Could you check a few things on this model? Use its own coordinates, in mm. Give positions to 0.01 mm unless a question says otherwise; leave off trailing zeros.
1. Imagine slicing it at A-A (z = 1.9). Count the separate pieces of the cut face and the enclosed holes in it, plus the area to 3 significant figures.
2. I need wall thicknesses on line 1 along Y through (x, z) = (-120, 2.35); line 2 along Y through (x, z) = (-25.5, 1.45); line 3 along Y through (x, z) = (-93.5, 1). Which ranges of each line are inside material? Lowest first, please.
3. Thinking about a two-plate mould opening in X: for faces 1 (the cylindrical face through (-124.305, -1.532, 1.479)), 2 (the flat face through (-2, 14, 0)), which applies, +X half, -X half, draft (parallel to the pull), parting line (faces both ways), or undercut?
```python
from build123d import *

# Parameters (mm, degrees)
F0_W     = 282
F0_H     = 122
F0_R     = 1.85
F0_R_2   = 4
F1_DEPTH = 3


with BuildPart() as f1:
    # F0 (on Top) → F1 (new body)
    with BuildSketch(Plane.XY):
        Rectangle(F0_W, F0_H)
        with Locations((-136, -56)):
            Circle(F0_R, mode=Mode.SUBTRACT)
        with Locations((-120, -56)):
            Circle(F0_R, mode=Mode.SUBTRACT)
        with Locations((-104, -56)):
            Circle(F0_R, mode=Mode.SUBTRACT)
        with Locations((-88, -56)):
            Circle(F0_R, mode=Mode.SUBTRACT)
        with Locations((-72, -56)):
            Circle(F0_R, mode=Mode.SUBTRACT)
        with Locations((-56, -56)):
            Circle(F0_R, mode=Mode.SUBTRACT)
        with Locations((-40, -56)):
            Circle(F0_R, mode=Mode.SUBTRACT)
        with Locations((-24, -56)):
            Circle(F0_R, mode=Mode.SUBTRACT)
        with Locations((-8, -56)):
            Circle(F0_R, mode=Mode.SUBTRACT)
        with Locations((-128, -8)):
            Circle(F0_R, mode=Mode.SUBTRACT)
        with Locations((-96, -8)):
            Circle(F0_R, mode=Mode.SUBTRACT)
        with Locations((-64, -8)):
            Circle(F0_R, mode=Mode.SUBTRACT)
        with Locations((-32, -8)):
            Circle(F0_R, mode=Mode.SUBTRACT)
        with Locations((8, -56)):
            Circle(F0_R, mode=Mode.SUBTRACT)
        with Locations((24, -56)):
            Circle(F0_R, mode=Mode.SUBTRACT)
        with Locations((40, -56)):
            Circle(F0_R, mode=Mode.SUBTRACT)
        with Locations((56, -56)):
            Circle(F0_R, mode=Mode.SUBTRACT)
        with Locations((72, -56)):
            Circle(F0_R, mode=Mode.SUBTRACT)
        with Locations((88, -56)):
            Circle(F0_R, mode=Mode.SUBTRACT)
        with Locations((104, -56)):
            Circle(F0_R, mode=Mode.SUBTRACT)
        with Locations((120, -56)):
            Circle(F0_R, mode=Mode.SUBTRACT)
        with Locations((136, -56)):
            Circle(F0_R, mode=Mode.SUBTRACT)
        with Locations((0, -8)):
            Circle(F0_R, mode=Mode.SUBTRACT)
        with Locations((32, -8)):
            Circle(F0_R, mode=Mode.SUBTRACT)
        with Locations((64, -8)):
            Circle(F0_R, mode=Mode.SUBTRACT)
        with Locations((96, -8)):
            Circle(F0_R, mode=Mode.SUBTRACT)
        with Locations((128, -8)):
            Circle(F0_R, mode=Mode.SUBTRACT)
        with Locations((-136, 0)):
            Circle(F0_R, mode=Mode.SUBTRACT)
        with Locations((-128, 0)):
            Circle(F0_R_2, mode=Mode.SUBTRACT)
        with Locations((-120, 0)):
            Circle(F0_R, mode=Mode.SUBTRACT)
        with Locations((-128, 8)):
            Circle(F0_R, mode=Mode.SUBTRACT)
        with Locations((-104, 0)):
            Circle(F0_R, mode=Mode.SUBTRACT)
        with Locations((-96, 0)):
            Circle(F0_R_2, mode=Mode.SUBTRACT)
        with Locations((-88, 0)):
            Circle(F0_R, mode=Mode.SUBTRACT)
        with Locations((-72, 0)):
            Circle(F0_R, mode=Mode.SUBTRACT)
        with Locations((-96, 8)):
            Circle(F0_R, mode=Mode.SUBTRACT)
        with Locations((-64, 0)):
            Circle(F0_R_2, mode=Mode.SUBTRACT)
        with Locations((-56, 0)):
            Circle(F0_R, mode=Mode.SUBTRACT)
        with Locations((-40, 0)):
            Circle(F0_R, mode=Mode.SUBTRACT)
        with Locations((-64, 8)):
            Circle(F0_R, mode=Mode.SUBTRACT)
        with Locations((-32, 0)):
            Circle(F0_R_2, mode=Mode.SUBTRACT)
        with Locations((-24, 0)):
            Circle(F0_R, mode=Mode.SUBTRACT)
        with Locations((-8, 0)):
            Circle(F0_R, mode=Mode.SUBTRACT)
        with Locations((-32, 8)):
            Circle(F0_R, mode=Mode.SUBTRACT)
        with Locations((-136, 56)):
            Circle(F0_R, mode=Mode.SUBTRACT)
        with Locations((-120, 56)):
            Circle(F0_R, mode=Mode.SUBTRACT)
        with Locations((-104, 56)):
            Circle(F0_R, mode=Mode.SUBTRACT)
        with Locations((-88, 56)):
            Circle(F0_R, mode=Mode.SUBTRACT)
        with Locations((-72, 56)):
            Circle(F0_R, mode=Mode.SUBTRACT)
        with Locations((-56, 56)):
            Circle(F0_R, mode=Mode.SUBTRACT)
        with Locations((-40, 56)):
            Circle(F0_R, mode=Mode.SUBTRACT)
        with Locations((-24, 56)):
            Circle(F0_R, mode=Mode.SUBTRACT)
        with Locations((-8, 56)):
            Circle(F0_R, mode=Mode.SUBTRACT)
        Circle(F0_R_2, mode=Mode.SUBTRACT)
        with Locations((8, 0)):
            Circle(F0_R, mode=Mode.SUBTRACT)
        with Locations((24, 0)):
            Circle(F0_R, mode=Mode.SUBTRACT)
        with Locations((32, 0)):
            Circle(F0_R_2, mode=Mode.SUBTRACT)
        with Locations((0, 8)):
            Circle(F0_R, mode=Mode.SUBTRACT)
        with Locations((32, 8)):
            Circle(F0_R, mode=Mode.SUBTRACT)
        with Locations((40, 0)):
            Circle(F0_R, mode=Mode.SUBTRACT)
        with Locations((56, 0)):
            Circle(F0_R, mode=Mode.SUBTRACT)
        with Locations((64, 0)):
            Circle(F0_R_2, mode=Mode.SUBTRACT)
        with Locations((64, 8)):
            Circle(F0_R, mode=Mode.SUBTRACT)
        with Locations((72, 0)):
            Circle(F0_R, mode=Mode.SUBTRACT)
        with Locations((88, 0)):
            Circle(F0_R, mode=Mode.SUBTRACT)
        with Locations((96, 0)):
            Circle(F0_R_2, mode=Mode.SUBTRACT)
        with Locations((104, 0)):
            Circle(F0_R, mode=Mode.SUBTRACT)
        with Locations((96, 8)):
            Circle(F0_R, mode=Mode.SUBTRACT)
        with Locations((120, 0)):
            Circle(F0_R, mode=Mode.SUBTRACT)
        with Locations((128, 0)):
            Circle(F0_R_2, mode=Mode.SUBTRACT)
        with Locations((136, 0)):
            Circle(F0_R, mode=Mode.SUBTRACT)
        with Locations((128, 8)):
            Circle(F0_R, mode=Mode.SUBTRACT)
        with Locations((8, 56)):
            Circle(F0_R, mode=Mode.SUBTRACT)
        with Locations((24, 56)):
            Circle(F0_R, mode=Mode.SUBTRACT)
        with Locations((40, 56)):
            Circle(F0_R, mode=Mode.SUBTRACT)
        with Locations((56, 56)):
            Circle(F0_R, mode=Mode.SUBTRACT)
        with Locations((72, 56)):
            Circle(F0_R, mode=Mode.SUBTRACT)
        with Locations((88, 56)):
            Circle(F0_R, mode=Mode.SUBTRACT)
        with Locations((104, 56)):
            Circle(F0_R, mode=Mode.SUBTRACT)
        with Locations((120, 56)):
            Circle(F0_R, mode=Mode.SUBTRACT)
        with Locations((136, 56)):
            Circle(F0_R, mode=Mode.SUBTRACT)
    extrude(amount=F1_DEPTH)


solid = f1.part
```
Derived:
1. separate pieces: 1
1. enclosed holes: 81
1. area: 33,200 mm2
2. line 1: y = -61 to -57.85, -54.15 to -1.85, 1.85 to 54.15, 57.85 to 61
2. line 2: y = -61 to -57.08, -54.92 to -1.08, 1.08 to 54.92, 57.08 to 61
2. line 3: y = -61 to -3.12, 3.12 to 61
3. face 1: undercut
3. face 2: draft
